Autodesk Inventor part; units mm, degrees
ref_plane "YZ Plane" through (0, 0, 0) normal (1, 0, 0) x (0, 1, 0)
ref_plane "XZ Plane" through (0, 0, 0) normal (0, 1, 0) x (-1, 0, 0)
ref_plane "XY Plane" through (0, 0, 0) normal (0, 0, 1) x (1, 0, 0)
sketch "Sketch1" plane through (0, 0, 0) normal (0, 0, 1) x (1, 0, 0)
  line L0 (5, 7.5) -> (2.5, 7.5)
  line L1 (0, 5) -> (0, -5)
  line L2 (2.5, -7.5) -> (5, -7.5)
  line L3 (5.5, -7) -> (5.5, 7)
  line L4 (2.1464, 7.3536) -> (0.1464, 5.3536)
  line L5 (2.1464, -7.3536) -> (0.1464, -5.3536)
  line L6 (5.5, 0) -> (-0.5, 0) construction
  arc A0 (5.5, 7) -> (5, 7.5) centre (5, 7) ccw
  arc A1 (5, -7.5) -> (5.5, -7) centre (5, -7) ccw
  arc A2 (2.1464, -7.3536) -> (2.5, -7.5) centre (2.5, -7) ccw
  arc A3 (0, -5) -> (0.1464, -5.3536) centre (0.5, -5) ccw
  arc A4 (0.1464, 5.3536) -> (0, 5) centre (0.5, 5) ccw
  arc A5 (2.5, 7.5) -> (2.1464, 7.3536) centre (2.5, 7) ccw
  line L7 (5, 7) -> (5, -7)
  line L8 (5, -7) -> (2.5, -7)
  line L9 (2.5, -7) -> (0.5, -5)
  line L10 (0.5, -5) -> (0.5, 5)
  line L11 (0.5, 5) -> (2.5, 7)
  line L12 (2.5, 7) -> (5, 7)
  line L13 (7.5, 13.5) -> (-10, 13.5)
  line L14 (-10, 13.5) -> (-10, -13.5)
  line L15 (-10, -13.5) -> (7.5, -13.5)
  line L16 (7.5, -13.5) -> (7.5, 13.5)
  line L17 (5.5, 0) -> (7.5, 0) construction
  point P0 (0, 0)
  point P1 (-0.5, 0)
  point P2 (5.5, 7.5)
  point P3 (5.5, -7.5)
  point P4 (-0.5, 0)
  point P5 (0, 0)
  dimension "d0" = 0.5
  dimension "d1" = 15
  dimension "d2" = 5.5
  dimension "d3" = 0.5
  dimension "d4" = 135
  dimension "d5" = 3
  dimension "d6" = 0.5
  dimension "d7" = 10
  dimension "d8" = 27
  dimension "d9" = 2
extrude "Extrusion1" add sketch "Sketch1" along normal blind 1 contours L16 L15 L14 L13
properties part number "P002-Cache-HDMI"
For this review, take the finished solid that the model builds, in its own axes (mm). A direction names the side the tool comes from. Round coordinates to 2 decimals unless told otherwise and drop trailing zeros. Write each loop counter-clockwise with the first axis right and the second up, starting at its lowest first coordinate (ties: lowest second). Pieces come first, ordered by that corner, then holes. Notation, with made-up numbers: M 89.25,-7 L 96.25,-7 A10 ccw 96.25,7 Z; hole C -2,33 d4. An arc over 180 degrees is marked long. One line per item, written item: value. Start each with the question number.
(1) Insertion check: pin 1 (1.5 mm diameter, centred on x = 1.5, y = -6.5, fed in from -Z). The pin has a flat end and moves straight along its axis. Give the tip position at first contact, or say it passes through.
(2) We need section B-B (z = 0.5). Give the boundary of the cut face in (x, y), and give its area (3 significant figures).
(3) Machinability: for faces 1 (the flat face through (1.16, 6.37, 0.49)), 2 (the flat face through (-10, 0.2, 0.5)), which of the approach directions +Z, -Z, +X, -X, +Y, -Y give a long, thin tool a straight path to every point of the face, cutting with its end or side? Answer none if there is none.
(4) We need section A-A (y = -3.25). Give the boundary of the cut face in (x, z), and give its area (3 significant figures).
(5) The part is to be moulded in two halves that separate along Y. For faces 3 (the flat face through (0, 0.1, 0.5)), 4 (the flat face through (-1, 0, 1)), 5 (the flat face through (-1.4, -13.5, 0.5)), say which applies: released by +Y, released by -Y, zero draft, split by the parting line, or undercut.
(6) We need section C-C (x = 1). Give the boundary of the cut face in (y, z).
(7) Wall thickness on line 1 (X direction, y = 4, z = 0.35); line 2 (Y direction, x = 4, z = 0.8); line 3 (Y direction, x = 1.5, z = 0.45): over which ranges is each line inside the solid? List them lowest first.
Result:
1. pin 1: z = 0
2. outline: M -10,-13.5 L 7.5,-13.5 L 7.5,13.5 L -10,13.5 Z; hole M 0,-5 A0.5 ccw 0.15,-5.35 L 2.15,-7.35 A0.5 ccw 2.5,-7.5 L 5,-7.5 A0.5 ccw 5.5,-7 L 5.5,7 A0.5 ccw 5,7.5 L 2.5,7.5 A0.5 ccw 2.15,7.35 L 0.15,5.35 A0.5 ccw 0,5 Z
2. area: 395 mm²
3. face 1: +Z, -Z
3. face 2: +Z, -Z, -X, +Y, -Y
4. outline: M -10,0 L 0,0 L 0,1 L -10,1 Z; M 5.5,0 L 7.5,0 L 7.5,1 L 5.5,1 Z
4. area: 12.0 mm²
5. face 3: undercut
5. face 4: zero draft
5. face 5: released by -Y
6. outline: M -13.5,0 L -6.21,0 L -6.21,1 L -13.5,1 Z; M 6.21,0 L 13.5,0 L 13.5,1 L 6.21,1 Z
7. line 1: -10 to 0, 5.5 to 7.5
7. line 2: -13.5 to -7.5, 7.5 to 13.5
7. line 3: -13.5 to -6.71, 6.71 to 13.5
